Geometry: final body of the model. Coordinates: model frame, mm. A direction names the side the tool comes from. Give positions to 0.01 mm unless a question says otherwise; leave off trailing zeros.
Q1. Pin query (flat end, axial travel): pin 1 (1.5 mm diameter, centred on x = 10.5, z = -27.5, fed in from +Y); pin 2 (3 mm diameter, centred on x = 11.38, z = 35.99, fed in from -Y); pin 3 (4 mm diameter, centred on x = 5.27, z = -34.1, fed in from +Y); pin 4 (12 mm diameter, centred on y = -1, z = 4, fed in from -X). Return the tip coordinate at first contact, or that it passes through.
Q2. Line query: L1, parallel to Z at x = 35.5, y = -11.25; L2, parallel to Z at x = -29.5, y = -7.75; L3, parallel to X at y = -3, z = 2. Output: solid intervals per line, ascending.
Q3. Cut plane A-A on y = -8.75. Count the separate pieces of the cut face and the enclosed holes in it, plus the area to 3 significant figures.
Q4. Reachability of faces 1 (the face through (38.553, -5.037, 3.052)), 2 (the face through (-24.79, 1.97, 24.82)) from +Z, -Z, +X, -X, +Y, -Y: full face, straight path, thin tool, end or side. Return the list, or none.
```python
from build123d import *

# Parameters (mm, degrees)
BOSS_EXTRUDE1_OUTLINE_R                              = 37
BOSS_EXTRUDE1_OUTLINE_R_2                            = 2.1
BOSS_EXTRUDE1_OUTLINE_R_3                            = 32
BOSS_EXTRUDE1_DEPTH                                  = 4
BOSS_EXTRUDE2_START                                  = -2
SKETCH2_R                                            = 37
SKETCH2_R_2                                          = 32
BOSS_EXTRUDE2_DEPTH                                  = 2
BOSS_EXTRUDE3_OUTLINE_W                              = 2
BOSS_EXTRUDE3_OUTLINE_H                              = 4
BOSS_EXTRUDE4_START                                  = 4
SKETCH4_R                                            = 37
SKETCH4_R_2                                          = 32.5
BOSS_EXTRUDE4_DEPTH                                  = 4
BOSS_EXTRUDE5_START                                  = 10
SKETCH5_R                                            = 40
SKETCH5_R_2                                          = 32.5
BOSS_EXTRUDE5_DEPTH                                  = 10
SKETCH6_R                                            = 40
SKETCH6_R_2                                          = 37
BOSS_EXTRUDE6_DEPTH                                  = 10
M3_CLEARANCE_HOLE1_D                                 = 3.4
SKETCH9_R                                            = 41.75
SKETCH9_R_2                                          = 40
BOSS_EXTRUDE7_DEPTH                                  = 20
CSK_FOR_M3_SOCKET_COUNTERSUNK_HEAD_SCREW_D           = 3.6
CSK_FOR_M3_SOCKET_COUNTERSUNK_HEAD_SCREW_CSINK_D     = 6.94
CSK_FOR_M3_SOCKET_COUNTERSUNK_HEAD_SCREW_CSINK_ANGLE = 90
SKETCH13_R                                           = 32
SKETCH13_R_2                                         = 30
BOSS_EXTRUDE8_DEPTH                                  = 2


# Read off the part's stored shape, not the designer's step: Boss-Extrude1, Boss-Extrude3
with BuildPart() as part:
    # Boss-Extrude1 outline → Boss-Extrude1 (new body)
    with BuildSketch(Plane(origin=(0, 0, 0), x_dir=(1, 0, 0), z_dir=(0, 1, 0))):
        Circle(BOSS_EXTRUDE1_OUTLINE_R)
        with Locations((-28.958107202, -18.753080475)):
            Circle(BOSS_EXTRUDE1_OUTLINE_R_2, mode=Mode.SUBTRACT)
        with Locations((-21.95036426, -26.616376704)):
            Circle(BOSS_EXTRUDE1_OUTLINE_R_2, mode=Mode.SUBTRACT)
        with Locations((-25.756086146, -22.953736656)):
            Circle(BOSS_EXTRUDE1_OUTLINE_R_2, mode=Mode.SUBTRACT)
        with Locations((-17.630144441, -29.655151441)):
            Circle(BOSS_EXTRUDE1_OUTLINE_R_2, mode=Mode.SUBTRACT)
        with Locations((-12.896688979, -31.998834563)):
            Circle(BOSS_EXTRUDE1_OUTLINE_R_2, mode=Mode.SUBTRACT)
        with Locations((-7.860946057, -33.592492124)):
            Circle(BOSS_EXTRUDE1_OUTLINE_R_2, mode=Mode.SUBTRACT)
        with Locations((-2.640949223, -34.398770141)):
            Circle(BOSS_EXTRUDE1_OUTLINE_R_2, mode=Mode.SUBTRACT)
        with Locations((-31.481374768, -14.112867982)):
            Circle(BOSS_EXTRUDE1_OUTLINE_R_2, mode=Mode.SUBTRACT)
        with Locations((-33.266745593, -9.141861826)):
            Circle(BOSS_EXTRUDE1_OUTLINE_R_2, mode=Mode.SUBTRACT)
        with Locations((-34.272372097, -3.956578176)):
            Circle(BOSS_EXTRUDE1_OUTLINE_R_2, mode=Mode.SUBTRACT)
        with Locations((2.640949223, -34.398770141)):
            Circle(BOSS_EXTRUDE1_OUTLINE_R_2, mode=Mode.SUBTRACT)
        with Locations((7.860946057, -33.592492124)):
            Circle(BOSS_EXTRUDE1_OUTLINE_R_2, mode=Mode.SUBTRACT)
        with Locations((12.896688979, -31.998834563)):
            Circle(BOSS_EXTRUDE1_OUTLINE_R_2, mode=Mode.SUBTRACT)
        with Locations((17.630144441, -29.655151441)):
            Circle(BOSS_EXTRUDE1_OUTLINE_R_2, mode=Mode.SUBTRACT)
        with Locations((21.95036426, -26.616376704)):
            Circle(BOSS_EXTRUDE1_OUTLINE_R_2, mode=Mode.SUBTRACT)
        with Locations((25.756086146, -22.953736656)):
            Circle(BOSS_EXTRUDE1_OUTLINE_R_2, mode=Mode.SUBTRACT)
        with Locations((28.958107202, -18.753080475)):
            Circle(BOSS_EXTRUDE1_OUTLINE_R_2, mode=Mode.SUBTRACT)
        with Locations((31.481374768, -14.112867982)):
            Circle(BOSS_EXTRUDE1_OUTLINE_R_2, mode=Mode.SUBTRACT)
        with Locations((33.266745593, -9.141861826)):
            Circle(BOSS_EXTRUDE1_OUTLINE_R_2, mode=Mode.SUBTRACT)
        with Locations((34.272372097, -3.956578176)):
            Circle(BOSS_EXTRUDE1_OUTLINE_R_2, mode=Mode.SUBTRACT)
        with Locations((-34.474683246, 1.321444312)):
            Circle(BOSS_EXTRUDE1_OUTLINE_R_2, mode=Mode.SUBTRACT)
        with Locations((-33.86893704, 6.568493266)):
            Circle(BOSS_EXTRUDE1_OUTLINE_R_2, mode=Mode.SUBTRACT)
        with Locations((-32.469331655, 11.661582305)):
            Circle(BOSS_EXTRUDE1_OUTLINE_R_2, mode=Mode.SUBTRACT)
        with Locations((-30.308672656, 16.481333739)):
            Circle(BOSS_EXTRUDE1_OUTLINE_R_2, mode=Mode.SUBTRACT)
        with Locations((-27.437604059, 20.914776678)):
            Circle(BOSS_EXTRUDE1_OUTLINE_R_2, mode=Mode.SUBTRACT)
        with Locations((-23.923421277, 24.857994979)):
            Circle(BOSS_EXTRUDE1_OUTLINE_R_2, mode=Mode.SUBTRACT)
        with Locations((-19.848493778, 28.218562946)):
            Circle(BOSS_EXTRUDE1_OUTLINE_R_2, mode=Mode.SUBTRACT)
        with Locations((-15.308334406, 30.917711715)):
            Circle(BOSS_EXTRUDE1_OUTLINE_R_2, mode=Mode.SUBTRACT)
        with Locations((-10.409360652, 32.892175526)):
            Circle(BOSS_EXTRUDE1_OUTLINE_R_2, mode=Mode.SUBTRACT)
        with Locations((-5.266400306, 34.09567462)):
            Circle(BOSS_EXTRUDE1_OUTLINE_R_2, mode=Mode.SUBTRACT)
        Circle(BOSS_EXTRUDE1_OUTLINE_R_3, mode=Mode.SUBTRACT)
        with Locations((34.474683246, 1.321444312)):
            Circle(BOSS_EXTRUDE1_OUTLINE_R_2, mode=Mode.SUBTRACT)
        with Locations((33.86893704, 6.568493266)):
            Circle(BOSS_EXTRUDE1_OUTLINE_R_2, mode=Mode.SUBTRACT)
        with Locations((32.469331655, 11.661582305)):
            Circle(BOSS_EXTRUDE1_OUTLINE_R_2, mode=Mode.SUBTRACT)
        with Locations((30.308672656, 16.481333739)):
            Circle(BOSS_EXTRUDE1_OUTLINE_R_2, mode=Mode.SUBTRACT)
        with Locations((0, 34.5)):
            Circle(BOSS_EXTRUDE1_OUTLINE_R_2, mode=Mode.SUBTRACT)
        with Locations((5.266400306, 34.09567462)):
            Circle(BOSS_EXTRUDE1_OUTLINE_R_2, mode=Mode.SUBTRACT)
        with Locations((15.308334406, 30.917711715)):
            Circle(BOSS_EXTRUDE1_OUTLINE_R_2, mode=Mode.SUBTRACT)
        with Locations((10.409360652, 32.892175526)):
            Circle(BOSS_EXTRUDE1_OUTLINE_R_2, mode=Mode.SUBTRACT)
        with Locations((27.437604059, 20.914776678)):
            Circle(BOSS_EXTRUDE1_OUTLINE_R_2, mode=Mode.SUBTRACT)
        with Locations((23.923421277, 24.857994979)):
            Circle(BOSS_EXTRUDE1_OUTLINE_R_2, mode=Mode.SUBTRACT)
        with Locations((19.848493778, 28.218562946)):
            Circle(BOSS_EXTRUDE1_OUTLINE_R_2, mode=Mode.SUBTRACT)
    extrude(amount=BOSS_EXTRUDE1_DEPTH)

    # Sketch2 → Boss-Extrude2 (add)
    with BuildSketch(Plane(origin=(0, 0, 0), x_dir=(1, 0, 0), z_dir=(0, 1, 0)).offset(BOSS_EXTRUDE2_START)):
        with Locations(Location((0, 0, 0), (0, 0, 270))):
            Circle(SKETCH2_R)
        with Locations(Location((0, 0, 0), (0, 0, 270))):
            Circle(SKETCH2_R_2, mode=Mode.SUBTRACT)
    extrude(amount=BOSS_EXTRUDE2_DEPTH)

    # Boss-Extrude3 outline → Boss-Extrude3 (revolve)
    with BuildSketch(Plane.XY):
        with Locations((31, 0)):
            Rectangle(BOSS_EXTRUDE3_OUTLINE_W, BOSS_EXTRUDE3_OUTLINE_H)
    revolve(axis=Axis((0, 0, 0), (0, 1, 0)))

    # Sketch4 → Boss-Extrude4 (add)
    with BuildSketch(Plane.XZ.offset(2).offset(BOSS_EXTRUDE4_START)):
        with Locations(Location((0, 0, 0), (0, 0, 270))):
            Circle(SKETCH4_R)
        with Locations(Location((0, 0, 0), (0, 0, 270))):
            Circle(SKETCH4_R_2, mode=Mode.SUBTRACT)
    extrude(amount=-BOSS_EXTRUDE4_DEPTH)

    # Sketch5 → Boss-Extrude5 (add)
    with BuildSketch(Plane.XZ.offset(6).offset(BOSS_EXTRUDE5_START)):
        with Locations(Location((0, 0, 0), (0, 0, 270))):
            Circle(SKETCH5_R)
        with Locations(Location((0, 0, 0), (0, 0, 270))):
            Circle(SKETCH5_R_2, mode=Mode.SUBTRACT)
    extrude(amount=-BOSS_EXTRUDE5_DEPTH)

    # Sketch6 → Boss-Extrude6 (add)
    with BuildSketch(Plane(origin=(0, -6, 0), x_dir=(1, 0, 0), z_dir=(0, 1, 0))):
        with Locations(Location((0, 0, 0), (0, 0, 270))):
            Circle(SKETCH6_R)
        Circle(SKETCH6_R_2, mode=Mode.SUBTRACT)
    extrude(amount=BOSS_EXTRUDE6_DEPTH)

    # M3 Clearance Hole1 (through all)
    with Locations(Plane(origin=(0, 4, 0), x_dir=(1, 0, 0), z_dir=(0, 1, 0))):
        with Locations((-14.111594462, 35.013217529), (2.889734295, 37.639233995), (14.111594462, 35.013217529), (24.018152198, 29.123716538), (31.686044836, 20.519675013), (36.400569453, 10.003051708), (37.722298335, -1.445928197), (35.528036811, -12.76013716), (30.022305891, -22.885009264), (21.718279423, -30.876833369), (11.389952597, -35.9907138), (0, -37.75), (-11.389952597, -35.9907138), (-21.718279423, -30.876833369), (-30.022305891, -22.885009264), (-35.528036811, -12.76013716), (-37.722298335, -1.445928197), (-36.400569453, 10.003051708), (-31.686044836, 20.519675013), (-24.018152198, 29.123716538)):
            Hole(M3_CLEARANCE_HOLE1_D / 2)

    # Sketch9 → Boss-Extrude7 (add)
    with BuildSketch(Plane(origin=(0, -16, 0), x_dir=(1, 0, 0), z_dir=(0, 1, 0))):
        with Locations(Location((0, 0, 0), (0, 0, 90))):
            Circle(SKETCH9_R)
        Circle(SKETCH9_R_2, mode=Mode.SUBTRACT)
    extrude(amount=BOSS_EXTRUDE7_DEPTH)

    # CSK for M3 socket countersunk head screw1 (through all)
    with Locations(Plane(origin=(0, -16, 0), x_dir=(-1, 0, 0), z_dir=(0, -1, 0))):
        with Locations((14.111594462, 35.013217529), (24.017656287, 29.124125506), (31.685346016, 20.520754075), (36.400058422, 10.004911138), (37.72239673, -1.443358912), (35.529123055, -12.757112327), (30.024643795, -22.881941897), (21.721959578, -30.874244478), (11.394855176, -35.989161917), (0.005785128, -37.749999557), (-11.383824076, -35.992652714), (-21.712495699, -30.88090074), (-30.017629142, -22.891143281), (-35.525211372, -12.768001292), (-37.721952573, -1.45492064), (-36.403123186, 9.993754165), (-31.691634074, 20.511041653), (-24.026581612, 29.116762802), (-14.12232524, 35.008890725), (-2.901911355, 37.638297125)):
            CounterSinkHole(CSK_FOR_M3_SOCKET_COUNTERSUNK_HEAD_SCREW_D / 2, CSK_FOR_M3_SOCKET_COUNTERSUNK_HEAD_SCREW_CSINK_D / 2, counter_sink_angle=CSK_FOR_M3_SOCKET_COUNTERSUNK_HEAD_SCREW_CSINK_ANGLE)

    # Sketch13 → Boss-Extrude8 (add)
    with BuildSketch(Plane(origin=(0, 2, 0), x_dir=(1, 0, 0), z_dir=(0, 1, 0))):
        Circle(SKETCH13_R)
        with Locations(Location((0, 0, 0), (0, 0, 90))):
            Circle(SKETCH13_R_2, mode=Mode.SUBTRACT)
    extrude(amount=BOSS_EXTRUDE8_DEPTH)


solid = part.part
```
Data:
1. pin 1: stops at y = 4
1. pin 2: passes through
1. pin 3: stops at y = 0
1. pin 4: stops at x = -41.75
2. L1: z = -21.97 to -11.55, -8.44 to 10.97, 14.57 to 21.97
2. L2: z = -29.54 to -13.64, 13.64 to 21.16, 24.6 to 29.54
2. L3: x = -41.7 to -39.43, -36.01 to -32.44, 32.44 to 36.01, 39.44 to 41.7
3. separate pieces: 1
3. enclosed holes: 21
3. area: 1,950 mm2
4. face 1: +Y, -Y
4. face 2: +Y
